The listing builds one solid part. Answer for the finished solid, in the listing's coordinates (mm). A direction names the side the tool comes from. Round coordinates to 2 decimals unless told otherwise and drop trailing zeros. Write each loop counter-clockwise with the first axis right and the second up, starting at its lowest first coordinate (ties: lowest second). Pieces come first, ordered by that corner, then holes. Notation, with made-up numbers: (82, 1) - (86, 1) arc R31 cw to (86, 30) - close; hole circle Ø3 at (-39.75, 55.5). An arc over 180 degrees is marked (long way). Use a Markdown table: item, result. Add a question column.
1) Determine the mould class of faces 1 (the cylindrical face through (-23.42, 1.15, 2.77)), 2 (the flat face through (-20.66, -2, 1)), 3 (the flat face through (-26, 0, 0)) for opening direction X: +X half, -X half, draft (parallel to the pull), parting line (faces both ways), or undercut.
2) A tool of negligible diameter and unlimited length cuts with its end or side. For faces 4 (the flat face through (26, 0, 0)), 5 (the flat face through (20.66, -2, 1)), from which of +Z, -Z, +X, -X, +Y, -Y can it reach the whole face along a straight path? Write none if from no direction.
3) Find the intervals of material crossed by probe 1 along X at (y, z) = (-0.75, -2.25); probe 2 along X at (y, z) = (2.5, 1.5); probe 3 along Z at (x, y) = (-7, -0.25), in increasing order. Write a range as from..to.
4) This flat-tipped pin is pushed along its axis until it touches: P1, Ø2, axis at x = 15.5, y = -1.5, coming from the +Z side. Where does it stop, or does it pass through?
5) A cutting plane is placed at A-A (x = 11). Give the vertices of the cut face in (y, z), then the cut area to 3 significant figures.
```python
from build123d import *

# Parameters (mm, degrees)
ESQUISSE1_W     = 52
ESQUISSE1_H     = 3
CHANFREIN1_SIZE = 0.5
ESQUISSE3_W     = 0.74
ESQUISSE3_H     = 1


with BuildPart() as part:
    # Esquisse1 → Révolution1 (revolve)
    with BuildSketch(Plane.XY, mode=Mode.PRIVATE) as r_volution1_sk:
        with Locations((0, 1.5)):
            Rectangle(ESQUISSE1_W, ESQUISSE1_H)
    revolve(r_volution1_sk.sketch.rotate(Axis((0, 0, 0), (1, 0, 0)), 90), axis=Axis((0, 0, 0), (1, 0, 0)))

    # Chanfrein1
    chanfrein1_edges = [part.edges().sort_by_distance(p)[0] for p in [
        (26, 0, -3),
        (-26, 0, -3),
    ]]
    chamfer(chanfrein1_edges, length=CHANFREIN1_SIZE)

    # Esquisse3 → Enlèvement de matière-Révolution1 (revolve, cut)
    with BuildSketch(Plane.XY):
        with Locations((-21.03, 2.5)):
            Rectangle(ESQUISSE3_W, ESQUISSE3_H)
        with Locations((21.03, 2.5)):
            Rectangle(ESQUISSE3_W, ESQUISSE3_H)
    revolve(axis=Axis((0, 0, 0), (-1, 0, 0)), mode=Mode.SUBTRACT)


solid = part.part
```
Entries:
| question | item | result |
|---|---|---|
| 1 | face 1 | draft |
| 1 | face 2 | undercut |
| 1 | face 3 | -X half |
| 2 | face 4 | +Z, -Z, +X, +Y, -Y |
| 2 | face 5 | none |
| 3 | probe 1 | x = -26..-21.4, -20.66..20.66, 21.4..26 |
| 3 | probe 2 | x = -25.58..-21.4, -20.66..20.66, 21.4..25.58 |
| 3 | probe 3 | z = -2.99..2.99 |
| 4 | P1 | stops at z = 2.96 |
| 5 | outline | circle Ø6 at (0, 0) |
| 5 | area | 28.3 mm² |
